Verification items for the finished model (mm, model axes). Face numbers are marked on the shaded views. A direction names the side the tool comes from. Round coordinates to 2 decimals unless told otherwise and drop trailing zeros. Order: outer loops, then holes, each group sorted by start corner. A loop starts at its lowest first (then second) coordinate and runs counter-clockwise, first axis right, second up. Notation, with made-up numbers: (69.25, -18.75) -> (81.25, -18.75) arc R6 ccw to (81.25, -14.75) -> close; hole circle Ø5 at (58, 64.5). An arc over 180 degrees is marked (long way). Return JSON: item names as keys, results as strings. Group by question number.
1) Scan lines: L1, parallel to Y at x = 0, z = 56.8; L2, parallel to Y at x = 21, z = 51.5; L3, parallel to X at y = -2.5, z = 45.25. Record each from-to range of solid material in increasing order.
2) Depth check by flat-ended pin: pin 1 (3 mm diameter, centred on x = 12.5, y = -13.5, fed in from +Z); pin 2 (4 mm diameter, centred on x = -25.5, y = -7, fed in from -Z); pin 3 (3 mm diameter, centred on x = 23.67, z = 50.75, fed in from -Y); pin 4 (10 mm diameter, centred on y = -13, z = 61.5, fed in from -X). Enter the tip coordinate at first touch or a pass-through.
3) Tool access check on the marked faces 1 and 2. Record the directions out of +Z, -Z, +X, -X, +Y, -Y that give a thin tool (end or side, any length) a straight path to the whole face; none if there is none.
4) Section check C-C on x = 14.5. Enter the section's corners in (y, z).
5) Draft check along Z on the marked faces 3, 4 and 5. Enter one of: pulls with the +Z half, pulls with the -Z half, needs draft (parallel to the pull), parting line crosses it, or undercut.
6) Section check D-D on z = 56.5. State how many separate pieces and enclosed holes the cut face has, plus the area to 3 significant figures.
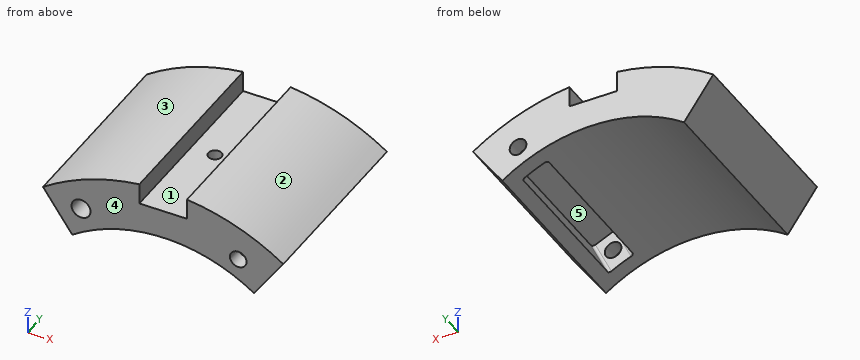
```python
from build123d import *

# Parameters (mm, degrees)
F3_DEPTH  = 60
F9_D      = 6
F9_DEPTH  = 35
F9_TIP    = 1.8025818571
F10_D     = 4.2
F10_DEPTH = 4.8
F10_TIP   = 1.2618073
F11_DEPTH = 12
F12_D     = 5.25


# Not quite as in the source:
# - a feature of the source that left no trace in its solid (it failed there, or was rolled back) is left out
# - a feature names something its author has since deleted; it is built from what else it names


with BuildPart() as f3:
    # F2 (on Front) → F3 (new body)
    with BuildSketch(Plane.XZ):
        with BuildLine():
            ThreePointArc((-28.634656432, 40.894527507), (0, 49.923), (28.634656432, 40.894527507))
            Line((28.634656432, 40.894527507), (37.8560447992, 54.0640349231))
            ThreePointArc((37.8560447992, 54.0640349231), (23.3966615381, 61.7138252653), (7.5, 65.5724789832))
            Line((7.5, 65.5724789832), (7.5, 59))
            Line((7.5, 59), (0, 59))
            Line((0, 59), (-7.5, 59))
            Line((-7.5, 59), (-7.5, 65.5724789832))
            ThreePointArc((-7.5, 65.5724789832), (-23.3966615381, 61.7138252653), (-37.8560447992, 54.0640349231))
            Line((-37.8560447992, 54.0640349231), (-28.634656432, 40.894527507))
        make_face()
    extrude(amount=F3_DEPTH)

    # F9
    with Locations(Plane.XZ.offset(60)):
        with Locations((-25.8774584852, 50.7873718787)):
            Hole(F9_D / 2, depth=F9_DEPTH)
            with Locations((0, 0, -(F9_DEPTH + F9_TIP / 2))):  # 118° drill point
                Cone(0, F9_D / 2, F9_TIP, mode=Mode.SUBTRACT)

    # F10
    with Locations(Plane.XY.offset(59)):
        with Locations((0, -30)):
            Hole(F10_D / 2, depth=F10_DEPTH)
            with Locations((0, 0, -(F10_DEPTH + F10_TIP / 2))):  # 118° drill point
                Cone(0, F10_D / 2, F10_TIP, mode=Mode.SUBTRACT)

    # F7 (on line) → F11 (cut)
    with BuildSketch(Plane(origin=(21.0180858076, 0, 45.0734304703), x_dir=(0.906307787, 0, -0.4226182617), z_dir=(0.4226182617, 0, 0.906307787))):
        with BuildLine():
            Line((0, -5), (0, -55))
            Line((0, -55), (3.487631816, -55))
            ThreePointArc((3.487631816, -55), (4.1947385971, -54.7071067812), (4.487631816, -54))
            Line((4.487631816, -54), (4.487631816, -6))
            ThreePointArc((4.487631816, -6), (4.1947385971, -5.2928932188), (3.487631816, -5))
            Line((3.487631816, -5), (0, -5))
        make_face()
        with BuildLine():
            Line((-3.359387327, -55), (0, -55))
            Line((0, -55), (0, -5))
            Line((0, -5), (-3.359387327, -5))
            ThreePointArc((-3.359387327, -5), (-4.0664941082, -5.2928932188), (-4.359387327, -6))
            Line((-4.359387327, -6), (-4.359387327, -54))
            ThreePointArc((-4.359387327, -54), (-4.0664941082, -54.7071067812), (-3.359387327, -55))
        make_face()
    extrude(amount=F11_DEPTH, mode=Mode.SUBTRACT)

    # F12 (through all)
    with Locations(Plane.XZ.offset(60)):
        with Locations((23.6666226575, 50.7532360741)):
            Hole(F12_D / 2)


solid = f3.part
```
Check result:
{
 "1": {"L1": "-60 to -32.1, -27.9 to 0", "L2": "-60 to -55, -5 to 0", "L3": "-31.68 to -21.09, 21.09 to 31.68"},
 "2": {"pin 1": "z = 65.08", "pin 2": "z = 41.67", "pin 3": "through", "pin 4": "x = -34.11"},
 "3": {"face 1": "+Z, +Y, -Y", "face 2": "+Z, +X, +Y, -Y"},
 "4": {"outline": "(-60, 47.77) -> (0, 47.77) -> (0, 64.39) -> (-60, 64.39) -> close"},
 "5": {"face 3": "pulls with the +Z half", "face 4": "needs draft", "face 5": "undercut"},
 "6": {"separate pieces": "1", "enclosed holes": "2", "area": "3,910 mm^2"}
}
